Geometry: final body of the model. Coordinates: model frame, mm. A direction names the side the tool comes from. Give positions to 0.01 mm unless a question says otherwise; leave off trailing zeros. Write each loop counter-clockwise with the first axis right and the second up, starting at its lowest first coordinate (ties: lowest second). Pieces come first, ordered by that corner, then holes. Notation, with made-up numbers: (31, 60.5) -> (73, 60.5) arc R16 cw to (73, 75.5) -> close; hole circle Ø8 at (43, -4.75). An arc over 180 degrees is marked (long way). Answer as a JSON object with one key per item and string values.
from build123d import *

# Parameters (mm, degrees)
BOSS_EXTRUDE1_DEPTH         = 63.5
M5_CLEARANCE_HOLE1_D        = 5.5
M5_CLEARANCE_HOLE2_D        = 5.5
M5_CLEARANCE_HOLE3_D        = 5.5
M5_CLEARANCE_HOLE4_D        = 5.5
F_23_0_154_DIAMETER_HOLE1_D = 3.9116
M5_CLEARANCE_HOLE5_D        = 5.5


with BuildPart() as part:
    # Sketch1 → Boss-Extrude1 (new body)
    with BuildSketch(Plane.XY):
        Polygon((0, 0), (0, 37.338), (23.114, 37.338), (23.114, 34.163), (3.302, 34.163), (3.302, 0), align=None)
    extrude(amount=BOSS_EXTRUDE1_DEPTH)

    # M5 Clearance Hole1 (through all)
    with Locations(Plane.ZY):
        with Locations((55.84134748, 24.208221519)):
            Hole(M5_CLEARANCE_HOLE1_D / 2)

    # M5 Clearance Hole2 (through all)
    with Locations(Plane.ZY):
        with Locations((7.677638483, 24.208221519)):
            Hole(M5_CLEARANCE_HOLE2_D / 2)

    # M5 Clearance Hole3 (through all)
    with Locations(Plane(origin=(0, 37.338, 0), x_dir=(1, 0, 0), z_dir=(0, 1, 0))):
        with Locations((13.368582087, -31.75)):
            Hole(M5_CLEARANCE_HOLE3_D / 2)

    # M5 Clearance Hole4 (through all)
    with Locations(Plane(origin=(0, 37.338, 0), x_dir=(1, 0, 0), z_dir=(0, 1, 0))):
        with Locations((13.368582087, -55.713693276)):
            Hole(M5_CLEARANCE_HOLE4_D / 2)

    # #23 (0.154) Diameter Hole1 (through all)
    with Locations(Plane.ZY):
        with Locations((39.767961445, 8.161533304), (23.72660366, 8.142354774), (23.72660366, 24.147573359), (39.720778954, 24.147573359)):
            Hole(F_23_0_154_DIAMETER_HOLE1_D / 2)

    # M5 Clearance Hole5 (through all)
    with Locations(Plane(origin=(0, 37.338, 0), x_dir=(1, 0, 0), z_dir=(0, 1, 0))):
        with Locations((13.368582087, -7.610649616)):
            Hole(M5_CLEARANCE_HOLE5_D / 2)


solid = part.part
Q1. Cut plane A-A (z = 31.75). Return the cut outline in (x, y), and give its area (3 significant figures).
Values:
{"outline": "(0, 0) -> (3.3, 0) -> (3.3, 34.16) -> (10.62, 34.16) -> (10.62, 37.34) -> (0, 37.34) -> close; (16.12, 34.16) -> (23.11, 34.16) -> (23.11, 37.34) -> (16.12, 37.34) -> close", "area": "169 mm²"}
Q2. Cut plane C-C (z = 6). Return the cut outline in (x, y), and give its area (3 significant figures).
Values:
{"outline": "(0, 0) -> (3.3, 0) -> (3.3, 22.03) -> (0, 22.03) -> close; (0, 26.39) -> (3.3, 26.39) -> (3.3, 34.16) -> (11.14, 34.16) -> (11.14, 37.34) -> (0, 37.34) -> close; (15.6, 34.16) -> (23.11, 34.16) -> (23.11, 37.34) -> (15.6, 37.34) -> close", "area": "158 mm²"}
Q3. Material intervals for L1, parallel to Z at x = 2, y = 25; L2, parallel to X at y = 19, z = 52.5; L3, parallel to Y at x = 4.25, z = 55, sorted ascending. Write a range as from..to.
Values:
{"L1": "0..5.04, 10.31..21.97, 25.49..37.96, 41.48..53.21, 58.47..63.5", "L2": "0..3.3", "L3": "34.16..37.34"}
Q4. First-contact query: P1, Ø6.5, axis at y = 24.21, z = 7.68, coming from the +X side; P2, Ø1.5, axis at x = 8, z = 8, coming from the -Y side. Flat tips, straight axial feed; report the tip coordinate or a pass-through.
Values:
{"P1": "x = 3.3", "P2": "y = 34.16"}
Q5. Mould query, pull axis Z, two halves, no side actions, for faces 1 (the flat face through (3, 24, 63.5)), 2 (the flat face through (0, 18, 31)), 3 (the cylindrical face through (1.67, 22.96, 25.28)). Classes: pulls with the +Z half, pulls with the -Z half, needs draft (parallel to the pull), parting line crosses it, or undercut.
Values:
{"face 1": "pulls with the +Z half", "face 2": "needs draft", "face 3": "undercut"}
Q6. Cut plane D-D (z = 15). Return the cut outline in (x, y).
Values:
{"outline": "(0, 0) -> (3.3, 0) -> (3.3, 34.16) -> (23.11, 34.16) -> (23.11, 37.34) -> (0, 37.34) -> close"}
Q7. Cut plane B-B (x = 2). Return the cut outline in (y, z).
Values:
{"outline": "(0, 0) -> (37.34, 0) -> (37.34, 63.5) -> (0, 63.5) -> close; hole circle Ø3.91 at (8.14, 23.73); hole circle Ø3.91 at (8.16, 39.77); hole circle Ø5.5 at (24.21, 7.68); hole circle Ø5.5 at (24.21, 55.84); hole circle Ø3.91 at (24.15, 23.73); hole circle Ø3.91 at (24.15, 39.72)"}
Q8. Set-up query: faces 4 (the cylindrical face through (13.965, 35.728, 10.295)), 5 (the flat face through (18, 34.163, 31)). Return all of +Z, -Z, +X, -X, +Y, -Y with unobstructed straight access to the full face (end or side cutting, diameter ignored); none if empty.
Values:
{"face 4": "+Y, -Y", "face 5": "+Z, -Z, +X, -Y"}
